Study the drawing (mm; zero at the part's minimum x, y, z) and answer. Give positions to 0.01 mm unless a question says otherwise; leave off trailing zeros. Loops run counter-clockwise (first coordinate to the right, second up) from the corner with the lowest first, then second, coordinate; pieces in that order, holes last. Notation, with made-up numbers: M 2,-26 L 39,-26 A19 ccw 39,-2 Z; hole C -21,34.5 d8. An arc over 180 degrees is marked long. Return JSON: item names as keys, results as strings.
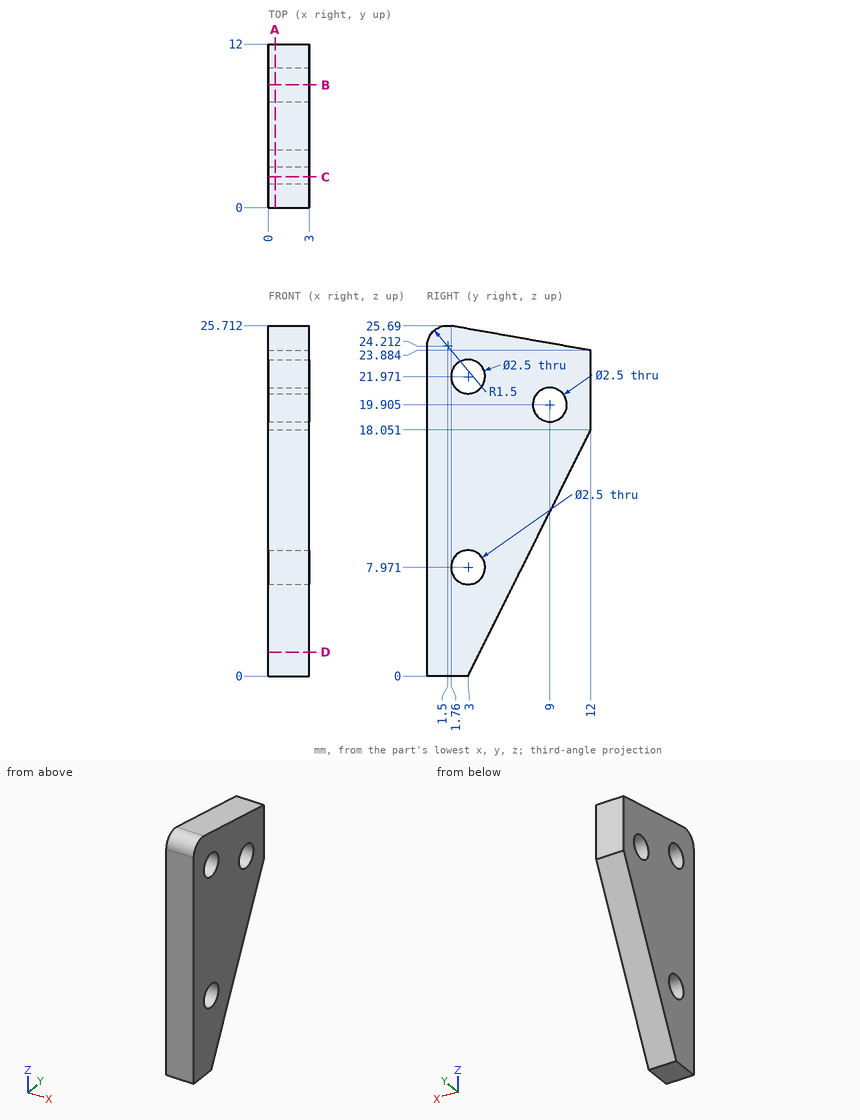
(1) The part is cut by section B-B (y = 9). Determine the outline of the cut face in (x, z) (1 decimal).
Values follow:
{"outline": "M 0,12 L 3,12 L 3,18.7 L 0,18.7 Z; M 0,21.2 L 3,21.2 L 3,24.4 L 0,24.4 Z"}
(2) Straight lines are drawn through the part: line 1 along Y through (x, z) = (1.45, 21) (1 decimal); line 2 along Y through (x, z) = (0.9, 20.5); line 3 along Y through (x, z) = (0.25, 7) (1 decimal). For each, find the intervals that lie inside material, in ascending order.
Values follow:
{"line 1": "0 to 2.2, 3.8 to 8.4, 9.6 to 12", "line 2": "0 to 7.9, 10.1 to 12", "line 3": "0 to 2.2, 3.8 to 6.5"}
(3) The part is cut by section C-C (y = 2.25). Determine the outline of the cut face in (x, z).
Values follow:
{"outline": "M 0,0 L 3,0 L 3,6.97 L 0,6.97 Z; M 0,8.97 L 3,8.97 L 3,20.97 L 0,20.97 Z; M 0,22.97 L 3,22.97 L 3,25.6 L 0,25.6 Z"}
(4) The part is cut by section A-A (x = 0.5). Give the number of separate pieces and of enclosed holes in the cut face, and give its area (3 significant figures).
Values follow:
{"separate pieces": "1", "enclosed holes": "3", "area": "203 mm²"}
(5) The part is cut by section D-D (z = 1.75). Determine the outline of the cut face in (x, y), and give its area (3 significant figures).
Values follow:
{"outline": "M 0,0 L 3,0 L 3,3.87 L 0,3.87 Z", "area": "11.6 mm²"}
